```python
from build123d import *

# Parameters (mm, degrees)
BOSS_EXTRUDE1_DEPTH     = 15
M2_5_CLEARANCE_HOLE1_D  = 2.9
CUT_EXTRUDE1_DEPTH      = 31.203476621
CUT_EXTRUDE1_DEPTH_BACK = 31.203476621
SKETCH3_R               = 4.365625
M2_CLEARANCE_HOLE1_D    = 2.4
SKETCH10_R              = 11.5
CUT_EXTRUDE3_DEPTH      = 1
CHAMFER1_SIZE           = 5.5
CHAMFER2_SIZE           = 7
FILLET1_R               = 5
FILLET2_R               = 5


with BuildPart() as part:
    # Sketch2 → Boss-Extrude1 (new, symmetric)
    with BuildSketch(Plane.XY):
        Polygon((0, 21.5), (0, -21.5), (19, -21.5), (19, -17), (4, -17), (4, 17), (19, 17), (19, 21.5), align=None)
    extrude(amount=BOSS_EXTRUDE1_DEPTH, both=True)

    # M2.5 Clearance Hole1 (through all)
    with Locations(Plane(origin=(0, -21.5, 0), x_dir=(-1, 0, 0), z_dir=(0, -1, 0))):
        with Locations((-14.5, -8), (-14.5, 8)):
            Hole(M2_5_CLEARANCE_HOLE1_D / 2)

    # Sketch3 → Cut-Extrude1 (cut, two sides: drawn at the far end of the back side and taken through both)
    with BuildSketch(Plane(origin=(4, 0, 0), x_dir=(0, 0, -1), z_dir=(1, 0, 0)).offset(-CUT_EXTRUDE1_DEPTH_BACK)):
        with Locations(Location((0, 0, 0), (0, 0, 90))):
            Circle(SKETCH3_R)
    extrude(amount=CUT_EXTRUDE1_DEPTH + CUT_EXTRUDE1_DEPTH_BACK, mode=Mode.SUBTRACT)

    # M2 Clearance Hole1 (through all)
    with Locations(Plane.ZY):
        with Locations((5.656854249, 5.656854249), (5.656854249, -5.656854249), (-5.656854249, -5.656854249), (-5.656854249, 5.656854249), (0, 0)):
            Hole(M2_CLEARANCE_HOLE1_D / 2)

    # Sketch10 → Cut-Extrude3 (cut)
    with BuildSketch(Plane.ZY):
        with Locations(Location((0, 0, 0), (0, 0, 270))):
            Circle(SKETCH10_R)
    extrude(amount=-CUT_EXTRUDE3_DEPTH, mode=Mode.SUBTRACT)

    # Chamfer1
    chamfer1_edges = [part.edges().sort_by_distance(p)[0] for p in [
        (4, 17, 0),
        (4, -17, 0),
    ]]
    chamfer(chamfer1_edges, length=CHAMFER1_SIZE)

    # Chamfer2
    chamfer2_edges = [part.edges().sort_by_distance(p)[0] for p in [
        (0, -21.5, 0),
        (0, 21.5, 0),
    ]]
    chamfer(chamfer2_edges, length=CHAMFER2_SIZE)

    # Fillet1
    fillet1_edges = [part.edges().sort_by_distance(p)[0] for p in [
        (19, -19.25, -15),
        (19, 19.25, 15),
        (19, -19.25, 15),
        (19, 19.25, -15),
    ]]
    fillet(fillet1_edges, radius=FILLET1_R)

    # Fillet2
    fillet2_edges = [part.edges().sort_by_distance(p)[0] for p in [
        (0, -14.5, 0),
        (0, 14.5, 0),
        (7, 21.5, 0),
        (7, -21.5, 0),
        (4, 11.5, 0),
        (4, -11.5, 0),
    ]]
    fillet(fillet2_edges, radius=FILLET2_R)


solid = part.part
```
The listing builds one solid part. Answer for the finished solid, in the listing's coordinates (mm). A direction names the side the tool comes from. Give positions to 0.01 mm unless a question says otherwise; leave off trailing zeros. Loops run counter-clockwise (first coordinate to the right, second up) from the corner with the lowest first, then second, coordinate; pieces in that order, holes last. Notation, with made-up numbers: (9.25, -7.5) - (49.25, -7.5) arc R32 ccw to (49.25, 30.5) - close; hole circle Ø11 at (-38, 5). An arc over 180 degrees is marked (long way). Return JSON: item names as keys, results as strings. Group by question number.
1. Find section A-A (x = 11). Write down the section's boundary in (y, z).
2. Determine the mould class of faces 4 (the flat face through (14, 17, 0)), 5 (the flat face through (3.5, 18, 0.2)), 6 (the cylindrical face through (15.839, 19.281, 8.555)) for opening direction Y: pulls with the +Y half, pulls with the -Y half, needs draft (parallel to the pull), parting line crosses it, or undercut.
3. Find section C-C (y = 0). Write down the section's boundary in (x, z).
4. Find section B-B (z = 0). Write down the section's boundary in (x, y).
5. Given pin 1 Ø4 at (y, z) = (-5.66, 5.66) entering from -X; pin 2 Ø2 at (y, z) = (-5.66, -5.66) entering from +X; pin 3 Ø1 at (x, z) = (13.5, 7) entering from +Y; pin 4 Ø2 at (y, z) = (-12.5, -6) entering from +X, each flat-ended and moving along its own axis, determine where each tip first touches the part or whether it passes through.
6. Straight lines are drawn through the part: line 1 (Y direction, x = 16.75, z = -13); line 2 (Y direction, x = 2, z = -6); line 3 (X direction, y = 9, z = 3). For each, find the intervals that lie inside material, in ascending order. Write a range as [from, to].
7. Which of the six approach directions +Z, -Z, +X, -X, +Y, -Y give full straight-line access (tool end or side, diameter ignored) to faces 1 (the flat face through (7.5, 15, -0.2)), 2 (the cylindrical face through (17, 19, -14)), 3 (the flat face through (1, -5, 0))?
8. Find section D-D (x = 14.5). Write down the section's boundary in (y, z).
Verdict:
{
 "1": {"outline": "(-21.5, -15) - (-17, -15) - (-17, 15) - (-21.5, 15) - close; (17, -15) - (21.5, -15) - (21.5, 15) - (17, 15) - close"},
 "2": {"face 4": "undercut", "face 5": "pulls with the +Y half", "face 6": "needs draft"},
 "3": {"outline": "(0, -15) - (4, -15) - (4, -4.37) - (1, -4.37) - (1, -11.5) - (0, -11.5) - close; (0, 11.5) - (1, 11.5) - (1, 4.37) - (4, 4.37) - (4, 15) - (0, 15) - close"},
 "4": {"outline": "(0, -12.43) arc R5 ccw to (1.46, -15.96) - (5.54, -20.04) arc R5 ccw to (9.07, -21.5) - (19, -21.5) - (19, -17) - (9.5, -17) - (5.46, -12.96) arc R5 cw to (4, -9.43) - (4, -4.37) - (1, -4.37) - (1, -11.5) - (0, -11.5) - close; (0, 11.5) - (1, 11.5) - (1, 4.37) - (4, 4.37) - (4, 9.43) arc R5 cw to (5.46, 12.96) - (9.5, 17) - (19, 17) - (19, 21.5) - (9.07, 21.5) arc R5 ccw to (5.54, 20.04) - (1.46, 15.96) arc R5 ccw to (0, 12.43) - close"},
 "5": {"pin 1": "stops at x = 1", "pin 2": "passes through", "pin 3": "stops at y = 21.5", "pin 4": "stops at x = 6"},
 "6": {"line 1": "y = [-21.5, -17], [17, 21.5]", "line 2": "y = [-16.5, -6.81], [-4.51, 4.51], [6.81, 16.5]", "line 3": "x = [1, 4]"},
 "7": {"face 1": "+Z, -Z, +X", "face 2": "-Z, +X, +Y, -Y", "face 3": "-X"},
 "8": {"outline": "(-21.5, -14.97) - (-17, -14.97) - (-17, -9.45) - (-21.5, -9.45) - close; (-21.5, -6.55) - (-17, -6.55) - (-17, 6.55) - (-21.5, 6.55) - close; (-21.5, 9.45) - (-17, 9.45) - (-17, 14.97) - (-21.5, 14.97) - close; (17, -14.97) - (21.5, -14.97) - (21.5, -9.45) - (17, -9.45) - close; (17, -6.55) - (21.5, -6.55) - (21.5, 6.55) - (17, 6.55) - close; (17, 9.45) - (21.5, 9.45) - (21.5, 14.97) - (17, 14.97) - close"}
}
